```python
from build123d import *

# Parameters (mm, degrees)
SKETCH_1_W        = 461.2
SKETCH_1_H        = 80.2
SKETCH_1_W_2      = 457.2
SKETCH_1_H_2      = 76.2
EXTRUDE_1_DEPTH   = 457.2
SKETCH_2_W        = 461.2
SKETCH_2_H        = 80.2
SKETCH_2_W_2      = 453.2
SKETCH_2_H_2      = 72.2
EXTRUDE_1_2_DEPTH = 2


with BuildPart() as part:
    # Эскиз1 → Extrude 1 (new body)
    with BuildSketch(Plane.XY):
        Rectangle(SKETCH_1_W, SKETCH_1_H)
        Rectangle(SKETCH_1_W_2, SKETCH_1_H_2, mode=Mode.SUBTRACT)
    extrude(amount=EXTRUDE_1_DEPTH)

    # Эскиз2 → Extrude 1 2 (add)
    with BuildSketch(Plane.XY.offset(457.2)):
        Rectangle(SKETCH_2_W, SKETCH_2_H)
        Rectangle(SKETCH_2_W_2, SKETCH_2_H_2, mode=Mode.SUBTRACT)
    extrude(amount=-EXTRUDE_1_2_DEPTH)


solid = part.part
```
For this review, take the finished solid that the model builds, in its own axes (mm). A direction names the side the tool comes from. Coordinates: 2 decimals unless noted, no trailing zeros. Loops run counter-clockwise (first coordinate to the right, second up) from the corner with the lowest first, then second, coordinate; pieces in that order, holes last. Notation, with made-up numbers: (-20, 31) - (24, 31) arc R27 ccw to (24, 49) - close; hole circle Ø4 at (28, 60). An arc over 180 degrees is marked (long way). Use one line per item in the form item = value. Start each with the question number.
1) Draft analysis for pull direction Y (two halves, no side actions). For faces 1 (the face through (-3, 40.1, 225)), 2 (the face through (-1, 39, 457.2)), 3 (the face through (-3, 38.1, 224)), state which applies: released by +Y, released by -Y, zero draft, split by the parting line, or undercut.
2) To check wall thickness, follow probe 1 along X at (y, z) = (-12, 375.5); probe 2 along Y at (x, z) = (102, 71.5). State the ranges of each line that lie inside material, in increasing order. Write a range as from..to.
3) Take a section at C-C (z = 165). State the section outline as (x, y) points, plus the area to 3 significant figures.
4) Take a section at A-A (y = 6). State the section outline as (x, z) points.
5) Take a section at B-B (x = 193). State the section outline as (y, z) points, plus the area to 3 significant figures.
6) For faces 4 (the face through (-228.6, -1, 224)), 5 (the face through (-230.6, -1, 225)), list the 3-axis set-ups (+Z, -Z, +X, -X, +Y, -Y) from which the entire face can be reached by the end or side of a thin tool; tool diameter is ignored.
From the geometry:
q1.face_1 = released by +Y
q1.face_2 = zero draft
q1.face_3 = undercut
q2.probe_1 = -230.6..-228.6, 228.6..230.6
q2.probe_2 = -40.1..-38.1, 38.1..40.1
q3.outline = (-230.6, -40.1) - (230.6, -40.1) - (230.6, 40.1) - (-230.6, 40.1) - close; hole (-228.6, -38.1) - (228.6, -38.1) - (228.6, 38.1) - (-228.6, 38.1) - close
q3.area = 2,150 mm2
q4.outline = (-230.6, 0) - (-228.6, 0) - (-228.6, 455.2) - (-226.6, 455.2) - (-226.6, 457.2) - (-230.6, 457.2) - close; (226.6, 455.2) - (228.6, 455.2) - (228.6, 0) - (230.6, 0) - (230.6, 457.2) - (226.6, 457.2) - close
q5.outline = (-40.1, 0) - (-38.1, 0) - (-38.1, 455.2) - (-36.1, 455.2) - (-36.1, 457.2) - (-40.1, 457.2) - close; (36.1, 455.2) - (38.1, 455.2) - (38.1, 0) - (40.1, 0) - (40.1, 457.2) - (36.1, 457.2) - close
q5.area = 1,840 mm2
q6.face_4 = -Z
q6.face_5 = +Z, -Z, -X, +Y, -Y
